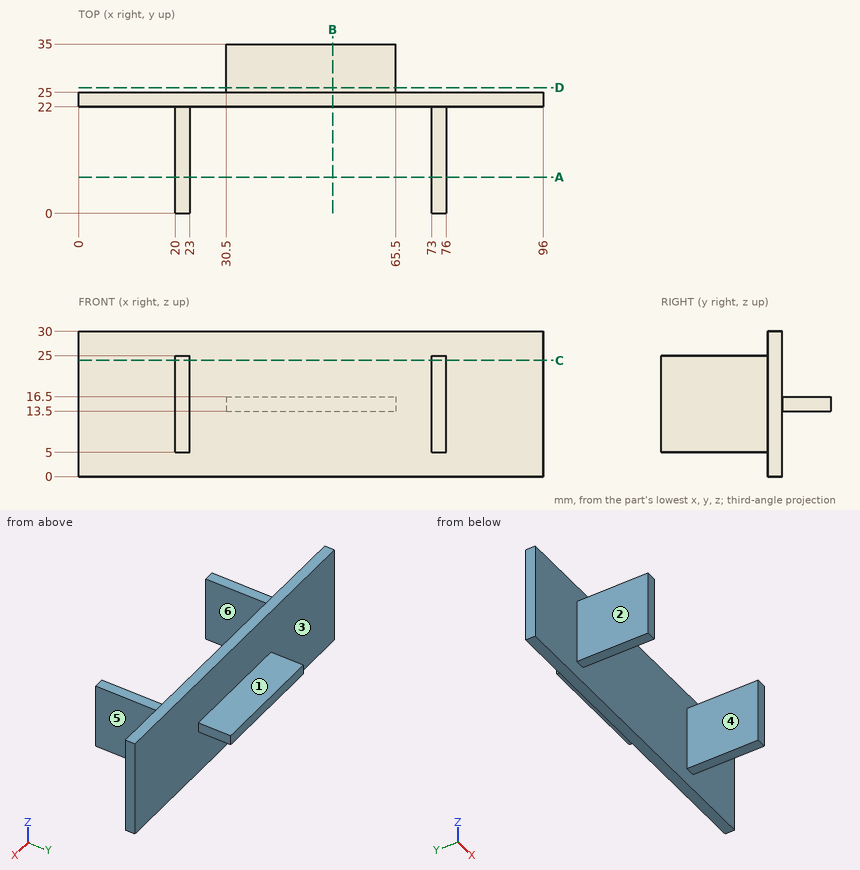
Source: three-view drawing plus pictorial views. Frame: mm from the lowest corner of the part. A direction names the side the tool comes from. Round coordinates to 2 decimals unless told otherwise and drop trailing zeros. Loops run counter-clockwise (first coordinate to the right, second up) from the corner with the lowest first, then second, coordinate; pieces in that order, holes last.
1. Section query C-C on z = 24. Output: boundary loops of the cut face in (x, y), and give its area (3 significant figures).
2. Ray query, L1, parallel to X at y = 5, z = 8.25; L2, parallel to Y at x = 74, z = 5.5; L3, parallel to Y at x = 15, z = 13.25. Return the intervals inside material, ascending.
3. Access query for the marked faces 1 and 2. Directions: +Z, -Z, +X, -X, +Y, -Y. A direction counts if a zero-diameter tool reaches every point of the face in a straight line with its end or side. Return the directions, or none.
4. Section query B-B on x = 52.5. Output: boundary loops of the cut face in (y, z), and give its area (3 significant figures).
5. Mould query, pull axis X, two halves, no side actions, for the marked faces 3, 4, 5 and 6. Classes: released by +X, released by -X, zero draft, split by the parting line, or undercut.
6. Section query A-A on y = 7.5. Output: boundary loops of the cut face in (x, z).
7. Section query D-D on y = 26. Output: boundary loops of the cut face in (x, z).
8. Contact query for flat-ended pins moving along their axis: pin 1 (3.5 mm diameter, centred on y = 29.5, z = 15, fed in from +X); pin 2 (5 mm diameter, centred on x = 42.5, y = 31.5, fed in from -Z); pin 3 (2.5 mm diameter, centred on x = 74, y = 15, fed in from +Z); pin 4 (15 mm diameter, centred on x = 25.5, z = 8.5, fed in from -Y). Output: stop coordinate, or through.
Answers below:
1. outline: (0, 22) - (20, 22) - (20, 0) - (23, 0) - (23, 22) - (73, 22) - (73, 0) - (76, 0) - (76, 22) - (96, 22) - (96, 25) - (0, 25) - close
1. area: 420 mm2
2. L1: x = 20 to 23, 73 to 76
2. L2: y = 0 to 25
2. L3: y = 22 to 25
3. face 1: +Z, +X, -X, +Y
3. face 2: +Z, -Z, -X, -Y
4. outline: (22, 0) - (25, 0) - (25, 13.5) - (35, 13.5) - (35, 16.5) - (25, 16.5) - (25, 30) - (22, 30) - close
4. area: 120 mm2
5. face 3: zero draft
5. face 4: undercut
5. face 5: released by +X
5. face 6: undercut
6. outline: (20, 5) - (23, 5) - (23, 25) - (20, 25) - close; (73, 5) - (76, 5) - (76, 25) - (73, 25) - close
7. outline: (30.5, 13.5) - (65.5, 13.5) - (65.5, 16.5) - (30.5, 16.5) - close
8. pin 1: stops at x = 65.5
8. pin 2: stops at z = 13.5
8. pin 3: stops at z = 25
8. pin 4: stops at y = 0
